Design review of the part built by this model. Coordinates are the model's own, in mm. Face numbers are marked on the shaded views. A direction names the side the tool comes from. Give positions to 0.01 mm unless a question says otherwise; leave off trailing zeros. Order: outer loops, then holes, each group sorted by start corner. A loop starts at its lowest first (then second) coordinate and runs counter-clockwise, first axis right, second up. Notation, with made-up numbers: (-26.5, -38.75) -> (8.5, -38.75) arc R20 cw to (8.5, -6.75) -> close; hole circle Ø2 at (9, 56). An arc over 180 degrees is marked (long way). Return JSON: item names as keys, results as strings.
```python
from build123d import *

# Parameters (mm, degrees)
BOX011_W                    = 20
BOX011_H                    = 2
BOX011_DEPTH                = 80
BOX012_W                    = 20
BOX012_H                    = 2
BOX012_DEPTH                = 80
COMPOUND005_PLACEMENT_ANGLE = 90
TUBE013_R                   = 10
TUBE013_R_2                 = 3.25
TUBE013_DEPTH               = 80
TUBE008_R                   = 7.625
TUBE008_R_2                 = 5.625
TUBE008_DEPTH               = 5
TUBE007_R                   = 7.625
TUBE007_R_2                 = 5.625
TUBE007_DEPTH               = 5
BOX005_W                    = 20
BOX005_H                    = 0.5
BOX005_DEPTH                = 40
BOX006_W                    = 20
BOX006_H                    = 0.5
BOX006_DEPTH                = 40
COMPOUND002_PLACEMENT_ANGLE = 90
TUBE006_R                   = 10
TUBE006_R_2                 = 3.25
TUBE006_DEPTH               = 40
CYLINDER002_R               = 5.625
CYLINDER002_DEPTH           = 100
CYLINDER001_R               = 12
CYLINDER001_DEPTH           = 6


with BuildPart() as cube011:
    # Box011 → Box011 (new body)
    with BuildSketch(Plane(origin=(-10, -1, -20), x_dir=(1, 0, 0), z_dir=(0, 0, 1))):
        with Locations((10, 1)):
            Rectangle(BOX011_W, BOX011_H)
    extrude(amount=BOX011_DEPTH)


with BuildPart() as fusion008:
    # Box012 → Box012 (new body)
    with BuildSketch(Plane(origin=(-10, -1, -20), x_dir=(1, 0, 0), z_dir=(0, 0, 1))):
        with Locations((10, 1)):
            Rectangle(BOX012_W, BOX012_H)
    extrude(amount=BOX012_DEPTH)


with BuildPart() as fusion008_1:
    # Compound005 placement: moved
    add(fusion008.part.rotate(Axis((0, 0, 0), (0, 0, 1)), COMPOUND005_PLACEMENT_ANGLE))

    # Fusion008: union Cube011
    add(cube011.part)


with BuildPart() as cut018:
    # Tube013 → Tube013 (new body)
    with BuildSketch(Plane.XY.offset(-20)):
        Circle(TUBE013_R)
        Circle(TUBE013_R_2, mode=Mode.SUBTRACT)
    extrude(amount=TUBE013_DEPTH)

    # Cut018: cut Fusion008
    add(fusion008_1.part, mode=Mode.SUBTRACT)


with BuildPart() as mountringgroove005:
    # Tube008 → Tube008 (new body)
    with BuildSketch(Plane.XY.offset(35)):
        Circle(TUBE008_R)
        Circle(TUBE008_R_2, mode=Mode.SUBTRACT)
    extrude(amount=TUBE008_DEPTH)


with BuildPart() as mountringgroove004:
    # Tube007 → Tube007 (new body)
    with BuildSketch(Plane.XY):
        Circle(TUBE007_R)
        Circle(TUBE007_R_2, mode=Mode.SUBTRACT)
    extrude(amount=TUBE007_DEPTH)


with BuildPart() as cube005:
    # Box005 → Box005 (new body)
    with BuildSketch(Plane(origin=(-10, -0.25, 0), x_dir=(1, 0, 0), z_dir=(0, 0, 1))):
        with Locations((10, 0.25)):
            Rectangle(BOX005_W, BOX005_H)
    extrude(amount=BOX005_DEPTH)


with BuildPart() as fusion002:
    # Box006 → Box006 (new body)
    with BuildSketch(Plane(origin=(-10, -0.25, 0), x_dir=(1, 0, 0), z_dir=(0, 0, 1))):
        with Locations((10, 0.25)):
            Rectangle(BOX006_W, BOX006_H)
    extrude(amount=BOX006_DEPTH)


with BuildPart() as fusion002_1:
    # Compound002 placement: moved
    add(fusion002.part.rotate(Axis((0, 0, 0), (0, 0, 1)), COMPOUND002_PLACEMENT_ANGLE))

    # Fusion002: union Cube005
    add(cube005.part)


with BuildPart() as cut011:
    # Tube006 → Tube006 (new body)
    with BuildSketch(Plane.XY):
        Circle(TUBE006_R)
        Circle(TUBE006_R_2, mode=Mode.SUBTRACT)
    extrude(amount=TUBE006_DEPTH)

    # Cut009: cut Fusion002
    add(fusion002_1.part, mode=Mode.SUBTRACT)

    # Cut010: cut MountringGroove004
    add(mountringgroove004.part, mode=Mode.SUBTRACT)

    # Cut011: cut MountringGroove005
    add(mountringgroove005.part, mode=Mode.SUBTRACT)


with BuildPart() as cut011_1:
    # Cut011 placement: moved
    add(cut011.part.moved(Location((0, 0, 7))))


with BuildPart() as cylinder002:
    # Cylinder002 → Cylinder002 (new body)
    with BuildSketch(Plane.XY):
        Circle(CYLINDER002_R)
    extrude(amount=CYLINDER002_DEPTH)


with BuildPart() as topring:
    # Cylinder001 → Cylinder001 (new body)
    with BuildSketch(Plane.XY.offset(42)):
        Circle(CYLINDER001_R)
    extrude(amount=CYLINDER001_DEPTH)

    # Cut008: cut Cylinder002
    add(cylinder002.part, mode=Mode.SUBTRACT)

    # Cut012: cut Cut011
    add(cut011_1.part, mode=Mode.SUBTRACT)


with BuildPart() as topring_1:
    # Cut012 placement: moved
    add(topring.part.moved(Location((0, 0, 4))))

    # Cut019: cut Cut018
    add(cut018.part, mode=Mode.SUBTRACT)


solid = topring_1.part
```
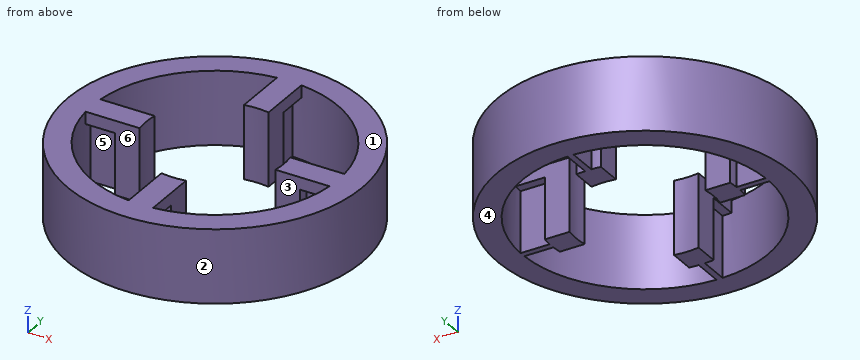
Item 1: Add section A-A (x = 3.25). Give the boundary of the cut face in (y, z), plus the area to 3 significant figures.
Result set:
{"outline": "(-11.55, 46) -> (-9.46, 46) -> (-9.46, 52) -> (-11.55, 52) -> close; (9.46, 46) -> (11.55, 46) -> (11.55, 52) -> (9.46, 52) -> close", "area": "25.1 mm^2"}
Item 2: Mouldability with a two-part tool opening along Y and no side actions: class the marked faces 1, 2 and 3 as released by +Y, released by -Y, zero draft, split by the parting line, or undercut.
Result set:
{"face 1": "zero draft", "face 2": "split by the parting line", "face 3": "undercut"}
Item 3: Add section D-D (y = -1.5). Give the boundary of the cut face in (x, z).
Result set:
{"outline": "(-11.91, 46) -> (-9.89, 46) -> (-9.89, 52) -> (-11.91, 52) -> close; (9.89, 46) -> (11.91, 46) -> (11.91, 52) -> (9.89, 52) -> close"}
Item 4: For pin 1 (1.2 mm diameter, centred on y = 8.5, z = 47.5, fed in from +X); pin 2 (1.2 mm diameter, centred on y = 8.5, z = 49.5, fed in from -X); pin 3 (1.2 mm diameter, centred on x = 8.5, z = 48.5, fed in from +Y), all flat-tipped, find the tip position at first contact; note any pin that passes through.
Result set:
{"pin 1": "stops at x = 9.03", "pin 2": "stops at x = -9.03", "pin 3": "stops at y = 9.03"}
Item 5: Add section C-C (y = -6.75). Give the boundary of the cut face in (x, z).
Result set:
{"outline": "(-9.92, 46) -> (-7.38, 46) -> (-7.38, 52) -> (-9.92, 52) -> close; (-1, 46) -> (1, 46) -> (1, 52) -> (-1, 52) -> close; (7.38, 46) -> (9.92, 46) -> (9.92, 52) -> (7.38, 52) -> close"}
Item 6: Wall thickness on L1, parallel to Y at x = -9.25, z = 46.95; L2, parallel to X at y = -7.5, z = 49.8; L3, parallel to X at y = -6.25, z = 48.25: over which ranges is each line inside the solid? List them lowest first. Write a range as [from, to].
Result set:
{"L1": "y = [-7.64, -3.8], [-0.25, 0.25], [3.8, 7.64]", "L2": "x = [-9.37, -6.61], [-1, 1], [6.61, 9.37]", "L3": "x = [-10.24, -7.81], [-1, 1], [7.81, 10.24]"}
Item 7: Machinability: for the marked faces 4, 5 and 6, which of the approach directions +Z, -Z, +X, -X, +Y, -Y give a long, thin tool a straight path to every point of the face, cutting with its end or side? Answer none if there is none.
Result set:
{"face 4": "-Z, +X, -X, +Y, -Y", "face 5": "-Z", "face 6": "+Z, -Z"}
